from build123d import *

# Parameters (mm, degrees)
F1_DEPTH = 55.626
F2_T     = -2.54
F3_R     = 15.24


with BuildPart() as f1:
    # F0 (on Top) → F1 (new body)
    with BuildSketch(Plane.XY):
        Polygon((-54.5444576688, -20.85977979), (54.5444576688, -20.85977979), (83.3149626851, 0), (54.5444576688, 20.85977979), (-54.5444576688, 20.85977979), (-77.8186991811, 0), align=None)
    extrude(amount=-F1_DEPTH)

    # F2
    f2_openings = [f1.faces().sort_by_distance(p)[0] for p in [
        (1.462281, 0, 0),
    ]]
    offset(amount=F2_T, openings=f2_openings)

    # F3
    f3_edges = [f1.edges().sort_by_distance(p)[0] for p in [
        (-63.792905, 9.15989, -53.086),
        (-63.792905, -9.15989, -53.086),
        (0.07388, -18.31978, -53.086),
        (66.354169, -9.15989, -53.086),
        (66.354169, 9.15989, -53.086),
        (0.07388, 18.31978, -53.086),
    ]]
    fillet(f3_edges, radius=F3_R)


solid = f1.part
CAD build for the part. Positions are in the model's coordinates, mm. A direction names the side the tool comes from. Round coordinates to 2 decimals unless told otherwise and drop trailing zeros. Write each loop counter-clockwise with the first axis right and the second up, starting at its lowest first coordinate (ties: lowest second). Pieces come first, ordered by that corner, then holes.
(1) Probe line 1 along Y through (x, z) = (35, -35); line 2 along X through (y, z) = (2, -10); line 3 along Y through (x, z) = (-34.5, -51.5). List the from-to ranges inside material, lowest first.
(2) Drop flat-ended pins along their axis: P1, Ø5, axis at x = 13, y = 0, coming from the +Z side; P2, Ø10, axis at y = 15, z = -47.5, coming from the -X side; P3, Ø1, axis at y = -16.5, z = -12, coming from the +X side. Give the stop position or say it passes through.
(3) Slice it at C-C, the plane z = -43.5. Write the cut outline in (x, y).
(4) Mould opens along X. For faces 3 (the face through (66.177, -9.288, -18.658)), 4 (the face through (-66.019, 10.576, -27.424)), 5 (the face through (69.131, 10.284, -27.424)) say: pulls with the +X half, pulls with the -X half, needs draft (parallel to the pull), parting line crosses it, or undercut.
(5) Slice it at B-B, the plane x = 21.5. Write the cut outline in (y, z).
(6) Slice it at A-A, the plane z = -32.5. Write the cut outline in (x, y), and give its area (3 significant figures).
(7) 3-axis set-ups, long thin cutter, end or side, ignore diameter. For faces 1 (the face through (-66.344, -10.284, -27.424)), 2 (the face through (-1, -18.32, -19)): which of +Z, -Z, +X, -X, +Y, -Y reach the whole face in a straight line?
From the geometry:
1. line 1: y = -20.86 to -18.32, 18.32 to 20.86
1. line 2: x = -75.59 to -71.78, 76.23 to 80.56
1. line 3: y = -20.86 to -9.85, 9.85 to 20.86
2. P1: stops at z = -53.09
2. P2: stops at x = -66.66
2. P3: stops at x = 61.25
3. outline: (-77.82, 0) - (-54.54, -20.86) - (54.54, -20.86) - (83.31, 0) - (54.54, 20.86) - (-54.54, 20.86) - close; hole (-72.38, 0) - (-53.16, -17.23) - (53.37, -17.23) - (77.13, 0) - (53.37, 17.23) - (-53.16, 17.23) - close
4. face 3: undercut
4. face 4: pulls with the -X half
4. face 5: pulls with the +X half
5. outline: (-20.86, -55.63) - (20.86, -55.63) - (20.86, 0) - (18.32, 0) - (18.32, -37.85) arc R15.24 cw to (3.08, -53.09) - (-3.08, -53.09) arc R15.24 cw to (-18.32, -37.85) - (-18.32, 0) - (-20.86, 0) - close
6. outline: (-77.82, 0) - (-54.54, -20.86) - (54.54, -20.86) - (83.31, 0) - (54.54, 20.86) - (-54.54, 20.86) - close; hole (-74.01, 0) - (-53.57, -18.32) - (53.72, -18.32) - (78.99, 0) - (53.72, 18.32) - (-53.57, 18.32) - close
6. area: 868 mm2
7. face 1: +Z, -Z, -X, -Y
7. face 2: +Z
